Source: CAD feature listing. Evaluate the final solid. Frame: model axes, mm. A direction names the side the tool comes from. Give positions to 0.01 mm unless a question says otherwise; leave off trailing zeros. Write each loop counter-clockwise with the first axis right and the second up, starting at its lowest first coordinate (ties: lowest second). Pieces come first, ordered by that corner, then holes. Notation, with made-up numbers: (73, -12.5) - (95, -12.5) arc R11 cw to (95, 7.5) - close; hole circle Ø8 at (65.25, -12). An arc over 180 degrees is marked (long way). One line per question, with ' | ' between items. Start each with the question number.
(1) Draft query along X for faces 3 (the cylindrical face through (19.699, -9.715, 2.014)), 4 (the cylindrical face through (-7.95, 0.65, 5.46)), 5 (the flat face through (-0.3, -9.5, 0.5)), 6 (the conical face through (-19.362, -9.355, 0.507)). Return one class per face: +X half, -X half, draft (parallel to the pull), parting line (faces both ways), or undercut.
(2) Ray query, line 1 (Z direction, x = -18, y = 6.25); line 2 (X direction, y = 1.25, z = 7); line 3 (Y direction, x = -10.5, z = 4.5). Return the intervals inside material, ascending. Write a range as [from, to].
(3) Pin query (flat end, axial travel): pin 1 (10 mm diameter, centred on x = 0, y = -1.5, fed in from +Z). Return the tip coordinate at first contact, or that it passes through.
(4) Access query for faces 1 (the cylindrical face through (7.85, 0.09, 5.46)), 2 (the flat face through (-10, 0, 8)). Directions: +Z, -Z, +X, -X, +Y, -Y. A direction counts if a zero-diameter tool reaches every point of the face in a straight line with its end or side. Return the directions, or none.
(5) Section C-C, the plane z = 4.25. Return loops of the section in (x, y), plus the area to 3 significant figures.
(6) Section A-A, the plane x = -10. Return loops of the section in (y, z), plus the area to 3 significant figures.
(7) Section B-B, the plane y = 0. Return loops of the section in (x, z), plus the area to 3 significant figures.
(8) Section D-D, the plane y = -7. Return loops of the section in (x, z), plus the area to 3 significant figures.
```python
from build123d import *

# Parameters (mm, degrees)
SKETCH1_W           = 40
SKETCH1_H           = 20
BOSS_EXTRUDE1_DEPTH = 3
SKETCH2_R           = 2.15
BOSS_EXTRUDE2_DEPTH = 5
FILLET1_R           = 1
CHAMFER1_SIZE       = 1


with BuildPart() as part:
    # Sketch1 → Boss-Extrude1 (new body)
    with BuildSketch(Plane.XY):
        Rectangle(SKETCH1_W, SKETCH1_H)
    extrude(amount=BOSS_EXTRUDE1_DEPTH)

    # Sketch2 → Boss-Extrude2 (add)
    with BuildSketch(Plane.XY.offset(3)):
        with Locations((10, 0)):
            Circle(SKETCH2_R)
        with Locations((-10, 0)):
            Circle(SKETCH2_R)
    extrude(amount=BOSS_EXTRUDE2_DEPTH)

    # Fillet1
    fillet1_edges = [part.edges().sort_by_distance(p)[0] for p in [
        (20, -10, 1.5),
        (-20, -10, 1.5),
        (-20, 10, 1.5),
        (20, 10, 1.5),
    ]]
    fillet(fillet1_edges, radius=FILLET1_R)

    # Chamfer1
    chamfer1_edges = [part.edges().sort_by_distance(p)[0] for p in [
        (20, 0, 0),
        (0, -10, 0),
        (-20, 0, 0),
        (0, 10, 0),
        (-19.707106781, 9.707106781, 0),
        (19.707106781, 9.707106781, 0),
        (-19.707106781, -9.707106781, 0),
        (19.707106781, -9.707106781, 0),
    ]]
    chamfer(chamfer1_edges, length=CHAMFER1_SIZE)


solid = part.part
```
Check sheet entries:
1) face 3: +X half | face 4: undercut | face 5: draft | face 6: -X half
2) line 1: [0, 3] | line 2: [-11.75, -8.25], [8.25, 11.75] | line 3: [-2.09, 2.09]
3) pin 1: z = 3
4) face 1: +Z | face 2: +Z, +X, -X, +Y, -Y
5) outline: circle Ø4.3 at (-10, 0); circle Ø4.3 at (10, 0) | area: 29.0 mm²
6) outline: (-10, 1) - (-9, 0) - (9, 0) - (10, 1) - (10, 3) - (2.15, 3) - (2.15, 8) - (-2.15, 8) - (-2.15, 3) - (-10, 3) - close | area: 80.5 mm²
7) outline: (-20, 1) - (-19, 0) - (19, 0) - (20, 1) - (20, 3) - (12.15, 3) - (12.15, 8) - (7.85, 8) - (7.85, 3) - (-7.85, 3) - (-7.85, 8) - (-12.15, 8) - (-12.15, 3) - (-20, 3) - close | area: 162 mm²
8) outline: (-20, 1) - (-19, 0) - (19, 0) - (20, 1) - (20, 3) - (-20, 3) - close | area: 119 mm²
